```python
from build123d import *


with BuildPart() as f3:
    # F0 (on Top) → F3 section 0
    with BuildSketch(Plane.XY, mode=Mode.PRIVATE) as f3_s0:
        Polygon((13.699032, 133.246349), (-67.237489, 115.85065), (-122.491575, 54.20394), (-130.958042, -28.146832), (-89.402989, -99.746472), (-13.699032, -133.246349), (67.237489, -115.85065), (122.491575, -54.20394), (130.958042, 28.146832), (89.402989, 99.746472), align=None)
    loft([Vertex(-2.990126, 0.499404, 254), f3_s0.sketch])


solid = f3.part
```
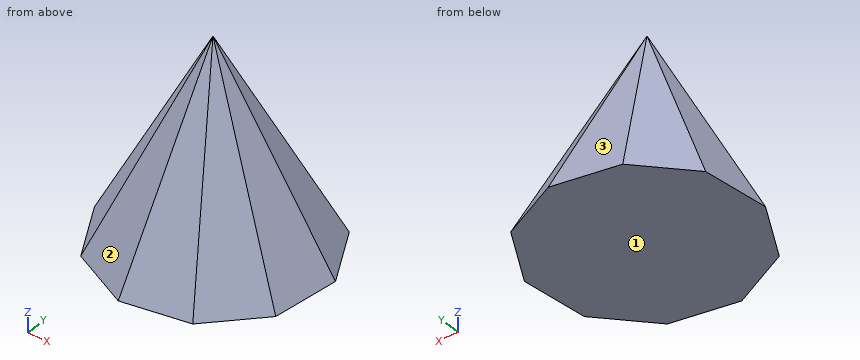
Geometry check sheet. Reference: the model listing, model coordinates, mm. Face numbers are marked on the shaded views. Give positions to 0.01 mm unless a question says otherwise; leave off trailing zeros. Write each loop counter-clockwise with the first axis right and the second up, starting at its lowest first coordinate (ties: lowest second). Pieces come first, ordered by that corner, then holes. Notation, with made-up numbers: (61.5, -17) - (76.5, -17) arc R11 ccw to (76.5, -12) - close; hole circle Ø8 at (81, 15.25). An arc over 180 degrees is marked (long way). Use a Markdown table: item, result.
Q1. Section check D-D, the plane z = 185. Enter the section's corners in (x, y), then the cut area to 3 significant figures.
Computed:
| item | result |
|---|---|
| outline | (-37.75, -7.28) - (-26.46, -26.73) - (-5.9, -35.83) - (16.09, -31.11) - (31.1, -14.36) - (33.4, 8.01) - (22.11, 27.46) - (1.54, 36.56) - (-20.44, 31.83) - (-35.45, 15.09) - close |
| area | 3,890 mm² |
Q2. Thickness scan on L1, parallel to X at y = 5.5, z = 77.5; L2, parallel to X at y = 53.5, z = 33; L3, parallel to Z at x = 20, y = -118.5. Record the ranges inside material, lowest first. Write a range as [from, to].
Computed:
| item | result |
|---|---|
| L1 | x = [-89.35, 88.63] |
| L2 | x = [-101.34, 96.76] |
| L3 | z = [0, 14.5] |
Q3. Draft check along Y on the marked faces 1, 2 and 3. Enter one of: pulls with the +Y half, pulls with the -Y half, needs draft (parallel to the pull), parting line crosses it, or undercut.
Computed:
| item | result |
|---|---|
| face 1 | needs draft |
| face 2 | pulls with the -Y half |
| face 3 | pulls with the +Y half |
Q4. Section check C-C, the plane y = 82. Enter the section's corners in (x, z), then the cut area to 3 significant figures.
Computed:
| item | result |
|---|---|
| outline | (-97.58, 0) - (99.7, 0) - (72.88, 45.42) - (7.26, 98.06) - (-48.38, 74.54) - close |
| area | 12,000 mm² |
Q5. Go/stop test with flat-tipped pins: P1, Ø1, axis at x = -45.5, z = 161.5, coming from the +Y side; P2, Ø6, axis at x = -57.5, y = 82, coming from the +Z side; P3, Ø5, axis at x = -33.5, z = 104.5, coming from the -Y side. Record where each tip stops, or that it passes through.
Computed:
| item | result |
|---|---|
| P1 | stops at y = 21.85 |
| P2 | stops at z = 66.83 |
| P3 | stops at y = -69.26 |
Q6. Section check A-A, the plane z = 147.5. Enter the section's corners in (x, y), then the cut area to 3 significant figures.
Computed:
| item | result |
|---|---|
| outline | (-56.65, -11.51) - (-39.22, -41.53) - (-7.48, -55.58) - (26.46, -48.29) - (49.62, -22.44) - (53.17, 12.09) - (35.75, 42.11) - (4.01, 56.16) - (-29.93, 48.87) - (-53.1, 23.02) - close |
| area | 9,270 mm² |
Q7. Section check B-B, the plane x = -43. Enter the section's corners in (y, z).
Computed:
| item | result |
|---|---|
| outline | (-120.28, 0) - (121.06, 0) - (72.33, 95.82) - (18.48, 168.96) - (-8.46, 174.59) - (-45.92, 136.4) - close |
